The listing builds one solid part. Answer for the finished solid, in the listing's coordinates (mm). A direction names the side the tool comes from. Coordinates: 2 decimals unless noted, no trailing zeros. Order: outer loops, then holes, each group sorted by start corner. A loop starts at its lowest first (then second) coordinate and runs counter-clockwise, first axis right, second up.
from build123d import *

# Parameters (mm, degrees)
SKETCH1_R               = 17.5
BOSS_EXTRUDE1_DEPTH     = 70
SKETCH4_W               = 50
SKETCH4_H               = 50
CUT_EXTRUDE1_DEPTH      = 731.855662905
CUT_EXTRUDE1_DEPTH_BACK = 650
SKETCH5_W               = 40
SKETCH5_H               = 40
SKETCH6_W               = 115
SKETCH6_H               = 55
SKETCH6_R               = 7
BOSS_EXTRUDE2_DEPTH     = 5
BOSS_EXTRUDE4_DEPTH     = 5
SKETCH13_R              = 7
CUT_EXTRUDE4_DEPTH      = 681.757849753
CUT_EXTRUDE5_DEPTH      = 681.757849753
CUT_EXTRUDE5_DEPTH_BACK = 681.757849753
SKETCH14_R              = 7


with BuildPart() as part:
    # Sketch1 → Boss-Extrude1 (new body)
    with BuildSketch(Plane.XY):
        Circle(SKETCH1_R)
    extrude(amount=BOSS_EXTRUDE1_DEPTH)

    # Sweep1: sweep along a path in Sketch3
    with BuildLine(Plane(origin=(0, 0, 0), x_dir=(1, 0, 0), z_dir=(0, 1, 0))) as sweep1_path:
        Line((0, 0), (0, 660))
    # Sketch4 → Sweep1 (sweep)
    with BuildSketch(Plane(origin=(0, 0, 0), x_dir=(-1, 0, 0), z_dir=(0, 0, -1))):
        Rectangle(SKETCH4_W, SKETCH4_H)
    sweep(path=sweep1_path.line)

    # Sketch5 → Cut-Extrude1 (cut, two sides: drawn at the far end of the back side and taken through both)
    with BuildSketch(Plane(origin=(0, 0, -660), x_dir=(-1, 0, 0), z_dir=(0, 0, -1)).offset(-CUT_EXTRUDE1_DEPTH_BACK)):
        Rectangle(SKETCH5_W, SKETCH5_H)
    extrude(amount=CUT_EXTRUDE1_DEPTH + CUT_EXTRUDE1_DEPTH_BACK, mode=Mode.SUBTRACT)

    # Sketch6 → Boss-Extrude2 (add)
    with BuildSketch(Plane(origin=(0, 0, -660), x_dir=(-1, 0, 0), z_dir=(0, 0, -1))):
        Rectangle(SKETCH6_W, SKETCH6_H)
        with Locations((-45, 0)):
            Circle(SKETCH6_R, mode=Mode.SUBTRACT)
        with Locations((45, 0)):
            Circle(SKETCH6_R, mode=Mode.SUBTRACT)
    extrude(amount=BOSS_EXTRUDE2_DEPTH)

    # Sketch12 → Boss-Extrude4 (add)
    with BuildSketch(Plane.ZY.offset(25)):
        with BuildLine():
            Line((-616.140431975, -25), (-656.140431975, -25))
            Line((-656.140431975, -25), (-656.140431975, -100))
            ThreePointArc((-656.140431975, -100), (-636.140431975, -120), (-616.140431975, -100))
            Line((-616.140431975, -100), (-616.140431975, -25))
        make_face()
    boss_extrude4 = extrude(amount=-BOSS_EXTRUDE4_DEPTH)

    # Sketch13 → Cut-Extrude4 (cut, through all)
    with BuildSketch(Plane.ZY.offset(25)):
        with Locations((-636.140431975, -100)):
            Circle(SKETCH13_R)
    cut_extrude4 = extrude(amount=-CUT_EXTRUDE4_DEPTH, mode=Mode.SUBTRACT)

    # Mirror1: Boss-Extrude4 across plane
    add(boss_extrude4.mirror(Plane(origin=(0, 0, 0), x_dir=(0, 0, 1), z_dir=(1, 0, 0))))

    # Mirror2: Cut-Extrude4 across plane
    add(cut_extrude4.mirror(Plane(origin=(0, 0, 0), x_dir=(0, 0, 1), z_dir=(1, 0, 0))), mode=Mode.SUBTRACT)

    # Sketch14 → Cut-Extrude5 (cut, two sides: drawn at the far end of the back side and taken through both)
    with BuildSketch(Plane(origin=(25, 0, 0), x_dir=(0, 0, -1), z_dir=(1, 0, 0)).offset(-CUT_EXTRUDE5_DEPTH_BACK)):
        with Locations((270, -2.5)):
            Circle(SKETCH14_R)
        with Locations((360, -2.5)):
            Circle(SKETCH14_R)
    extrude(amount=CUT_EXTRUDE5_DEPTH + CUT_EXTRUDE5_DEPTH_BACK, mode=Mode.SUBTRACT)


solid = part.part
1) Section A-A (x = 45) is taken. Give the vertices of the cut face in (y, z), then the cut area to 3 significant figures.
2) Determine the mould class of faces 1 (the face through (22.535, -119.995, -636.58)), 2 (the face through (0, 20, -330)), 3 (the face through (0, 0, -10)), 4 (the face through (-51.677, 2.103, -662.465)) for opening direction Z: released by +Z, released by -Z, zero draft, split by the parting line, or undercut.
3) Section B-B (z = -360) is taken. Give the vertices of the cut face in (x, y), then the cut area to 3 significant figures.
4) Section C-C (y = -82) is taken. Give the vertices of the cut face in (x, z).
5) Section D-D (z = -250.5) is taken. Give the vertices of the cut face in (x, y), then the cut area to 3 significant figures.
6) Each of these flat-tipped pins is pushed along its axis until it touches: P1, Ø4, axis at x = -23.5, y = -53, coming from the +Z side; P2, Ø5.5, axis at x = 11.5, z = -662, coming from the -Y side; P3, Ø8.5, axis at y = -2.5, z = -360, coming from the -X side; P4, Ø20, axis at y = -80, z = -626, coming from the +X side. Where does it stop, or does it pass through?
7) A tool of negligible diameter and unlimited length cuts with its end or side. For faces 5 (the face through (0, 25, -335)), 6 (the face through (-20, 0, -330)), 7 (the face through (-13.887, -10.648, 34.51)), 8 (the face through (25, -14, -408)), 9 (the face through (-25, -16, -408)), from which of +Z, -Z, +X, -X, +Y, -Y can it reach the whole face along a straight path? Write none if from no direction.
8) Consider L1, parallel to Y at x = 21, z = -270; L2, parallel to Z at x = 21.5, y = -2.5; L3, parallel to X at y = 16, z = -275. Determine where each line is inside the solid, lowest interval first.
Filled sheet:
1. outline: (-27.5, -665) - (-7, -665) - (-7, -660) - (-27.5, -660) - close; (7, -665) - (27.5, -665) - (27.5, -660) - (7, -660) - close
1. area: 205 mm2
2. face 1: split by the parting line
2. face 2: undercut
2. face 3: undercut
2. face 4: zero draft
3. outline: (-25, -25) - (25, -25) - (25, -9.5) - (20, -9.5) - (20, -20) - (-20, -20) - (-20, -9.5) - (-25, -9.5) - close; (-25, 4.5) - (-20, 4.5) - (-20, 20) - (20, 20) - (20, 4.5) - (25, 4.5) - (25, 25) - (-25, 25) - close
3. area: 760 mm2
4. outline: (-25, -656.14) - (-20, -656.14) - (-20, -616.14) - (-25, -616.14) - close; (20, -656.14) - (25, -656.14) - (25, -616.14) - (20, -616.14) - close
5. outline: (-25, -25) - (25, -25) - (25, 25) - (-25, 25) - close; hole (-20, -20) - (20, -20) - (20, 20) - (-20, 20) - close
5. area: 900 mm2
6. P1: stops at z = -616.14
6. P2: stops at y = -27.5
6. P3: passes through
6. P4: stops at x = 25
7. face 5: +Z, +X, -X, +Y
7. face 6: none
7. face 7: +Z
7. face 8: +Z, +X, +Y, -Y
7. face 9: +Z, -X, +Y, -Y
8. L1: y = -25 to -9.5, 4.5 to 25
8. L2: z = -665 to -367, -353 to -277, -263 to 0
8. L3: x = -25 to -20, 20 to 25
